Design review of the part built by this model. Coordinates are the model's own, in mm. Face numbers are marked on the shaded views. A direction names the side the tool comes from. Round coordinates to 2 decimals unless told otherwise and drop trailing zeros. Loops run counter-clockwise (first coordinate to the right, second up) from the corner with the lowest first, then second, coordinate; pieces in that order, holes last. Notation, with made-up numbers: M -18,51 L 41,51 A27 cw 41,89 Z; hole C 65,47.25 d8. An arc over 180 degrees is marked long. One line per item, written item: value. Start each with the question number.
Item 1: We need section B-B (x = -32). Write out the cut boundary in (y, z).
Item 2: We need section A-A (y = 36). Write out the cut boundary in (x, z).
Item 3: We need section C-C (x = 0). Write out the cut boundary in (y, z), then the cut area to 3 significant figures.
Item 4: We need section D-D (z = -1.5). State how many separate pieces and enclosed holes the cut face has, then the cut area to 3 significant figures.
Item 5: For line 1 along Y through (x, z) = (16, 0); line 2 along Z through (x, y) = (-32, 2); line 3 along X through (y, z) = (5, -2), list the stretches that pass through material, from the lowest coordinate up.
Item 6: For the marked faces 5, 6 and 7, list the 3-axis set-ups (+Z, -Z, +X, -X, +Y, -Y) from which the entire face can be reached by the end or side of a thin tool; tool diameter is ignored.
Item 7: Mouldability with a two-part tool opening along Y and no side actions: class the marked faces 1, 2, 3 and 4 as released by +Y, released by -Y, zero draft, split by the parting line, or undercut.
Item 8: Clearance check with flat-ended pins moving along their axes: pin 1 (4 mm diameter, centred on y = 24, z = 5.5, fed in from +X); pin 2 (6 mm diameter, centred on x = -35.5, z = -1.5, fed in from +Y); pin 3 (5.5 mm diameter, centred on y = 57.48, z = -0.33, fed in from +X); pin 4 (6.5 mm diameter, centred on y = 60, z = 1, fed in from -X). State where each tip first meets the part, or that it passes through.
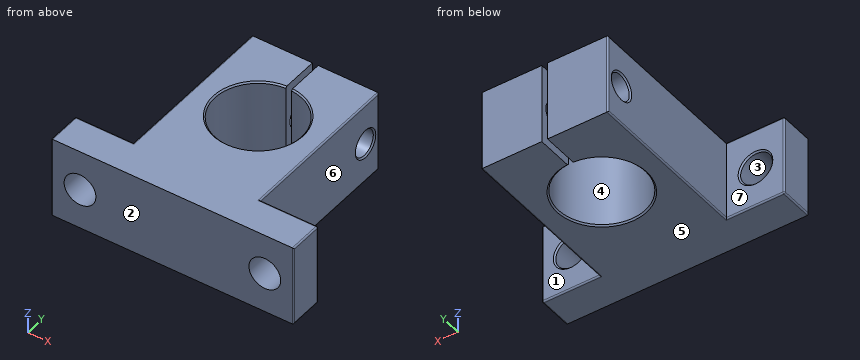
from build123d import *

# Parameters (mm, degrees)
BOSS_EXTRUDE1_DEPTH     = 14
SKETCH2_R               = 5.5
CUT_EXTRUDE1_DEPTH      = 73.965745388
CUT_EXTRUDE2_DEPTH      = 79.364532794
CUT_EXTRUDE2_DEPTH_BACK = 79.364532794
SKETCH5_R               = 4.5
CHAMFER2_SIZE           = 0.5
FILLET2_R               = 0.5


with BuildPart() as part:
    # Sketch1 → Boss-Extrude1 (new, symmetric)
    with BuildSketch(Plane.XY):
        with BuildLine():
            Line((-42, -6), (-42, 6))
            Line((-42, 6), (-22, 6))
            Line((-22, 6), (-22, 64))
            Line((-22, 64), (-1, 64))
            Line((-1, 64), (-1, 50.966629547))
            ThreePointArc((-1, 50.966629547), (0, 21), (1, 50.966629547))
            Line((1, 50.966629547), (1, 64))
            Line((1, 64), (22, 64))
            Line((22, 64), (22, 6))
            Line((22, 6), (42, 6))
            Line((42, 6), (42, -6))
            Line((42, -6), (-42, -6))
        make_face()
    extrude(amount=BOSS_EXTRUDE1_DEPTH, both=True)

    # Sketch2 → Cut-Extrude1 (cut, through all)
    with BuildSketch(Plane(origin=(0, 6, 0), x_dir=(1, 0, 0), z_dir=(0, 1, 0))):
        with Locations(Location((32, 0, 0), (0, 0, 180))):
            Circle(SKETCH2_R)
        with Locations(Location((-32, 0, 0), (0, 0, 180))):
            Circle(SKETCH2_R)
    extrude(amount=-CUT_EXTRUDE1_DEPTH, mode=Mode.SUBTRACT)

    # Sketch5 → Cut-Extrude2 (cut, two sides: drawn at the far end of the back side and taken through both)
    with BuildSketch(Plane(origin=(-1, 0, 0), x_dir=(0, 0, -1), z_dir=(1, 0, 0)).offset(-CUT_EXTRUDE2_DEPTH_BACK)):
        with Locations(Location((0.330734984, 57.483314774, 0), (0, 0, 90))):
            Circle(SKETCH5_R)
    extrude(amount=CUT_EXTRUDE2_DEPTH + CUT_EXTRUDE2_DEPTH_BACK, mode=Mode.SUBTRACT)

    # Chamfer2
    chamfer2_edges = [part.edges().sort_by_distance(p)[0] for p in [
        (0, 21, -14),
        (0, 21, 14),
        (37.5, 6, 0),
        (-26.5, 6, 0),
        (-22, 52.983314774, -0.330734984),
        (22, 52.983314774, -0.330734984),
    ]]
    chamfer(chamfer2_edges, length=CHAMFER2_SIZE)

    # Fillet2
    fillet2_edges = [part.edges().sort_by_distance(p)[0] for p in [
        (-32, 6, 14),
        (22, 35, -14),
        (32, 6, -14),
        (-42, 0, 14),
        (42, 0, -14),
        (-42, 0, -14),
        (-32, 6, -14),
        (-22, 35, -14),
        (42, 0, 14),
        (22, 64, 0),
        (42, 6, 0),
        (42, -6, 0),
        (-42, -6, 0),
        (-42, 6, 0),
        (-22, 64, 0),
        (32, 6, 14),
        (22, 35, 14),
        (-22, 35, 14),
    ]]
    fillet(fillet2_edges, radius=FILLET2_R)


solid = part.part
A:
1. outline: M -6,-14 L 5.5,-14 A0.5 ccw 6,-13.5 L 6,-6 L 5.5,-5.5 L -6,-5.5 Z; M -6,5.5 L 5.5,5.5 L 6,6 L 6,13.5 A0.5 ccw 5.5,14 L -6,14 Z
2. outline: M -22,-13.5 A0.5 ccw -21.5,-14 L -15.5,-14 L -15,-13.5 L -15,13.5 L -15.5,14 L -21.5,14 A0.5 ccw -22,13.5 Z; M 15,-13.5 L 15.5,-14 L 21.5,-14 A0.5 ccw 22,-13.5 L 22,13.5 A0.5 ccw 21.5,14 L 15.5,14 L 15,13.5 Z
3. outline: M -6,-14 L 20.5,-14 L 21,-13.5 L 21,13.5 L 20.5,14 L -6,14 Z
3. area: 756 mm2
4. separate pieces: 5
4. enclosed holes: 0
4. area: 2,210 mm2
5. line 1: -6 to 53, 61.97 to 64
5. line 2: -14 to -5.5, 5.5 to 14
5. line 3: -42 to -37.12, -26.88 to 26.88, 37.12 to 42
6. face 5: -Z, +X, -X, +Y, -Y
6. face 6: +Z, -Z, +X, +Y
6. face 7: +Z, -Z, -X, +Y
7. face 1: released by +Y
7. face 2: released by -Y
7. face 3: zero draft
7. face 4: undercut
8. pin 1: x = 22
8. pin 2: y = 6
8. pin 3: through
8. pin 4: x = -22
